from build123d import *

# Parameters (mm, degrees)
SKETCH1_R           = 2.1
SKETCH1_W           = 56
SKETCH1_H           = 115.35
SKETCH1_R_2         = 1.55
BOSS_EXTRUDE1_DEPTH = 3.175
FILLET1_R           = 4
SKETCH10_R          = 2.25
BOSS_EXTRUDE2_DEPTH = 3.175
CIRPATTERN4_COUNT   = 4


with BuildPart() as part:
    # Sketch1 → Boss-Extrude1 (new body)
    with BuildSketch(Plane.XY):
        Polygon((0, 163), (0, 0), (-163, 0), (-163, -17), (-180, -17), (-180, -123), (-163, -123), (-163, -140), (0, -140), (0, -303), (17, -303), (17, -320), (123, -320), (123, -303), (140, -303), (140, -140), (303, -140), (303, -123), (320, -123), (320, -17), (303, -17), (303, 0), (140, 0), (140, 163), (123, 163), (123, 180), (17, 180), (17, 163), align=None)
        with Locations((7.5, -277.5)):
            Circle(SKETCH1_R, mode=Mode.SUBTRACT)
        with Locations((30, -312.5)):
            Circle(SKETCH1_R, mode=Mode.SUBTRACT)
        with Locations((70, -312.5)):
            Circle(SKETCH1_R, mode=Mode.SUBTRACT)
        with Locations((22.5, -265)):
            Circle(SKETCH1_R, mode=Mode.SUBTRACT)
        with BuildLine():
            Line((51.95, -271), (51.95, -265))
            ThreePointArc((51.95, -265), (54, -262.95), (56.05, -265))
            Line((56.05, -265), (56.05, -271))
            ThreePointArc((56.05, -271), (54, -273.05), (51.95, -271))
        make_face(mode=Mode.SUBTRACT)
        with Locations((7.5, -242.5)):
            Circle(SKETCH1_R, mode=Mode.SUBTRACT)
        with Locations((7.5, -207.5)):
            Circle(SKETCH1_R, mode=Mode.SUBTRACT)
        with Locations((22.5, -240)):
            Circle(SKETCH1_R, mode=Mode.SUBTRACT)
        with Locations((70, -202.325)):
            Rectangle(SKETCH1_W, SKETCH1_H, mode=Mode.SUBTRACT)
        with Locations((-172.5, -110)):
            Circle(SKETCH1_R, mode=Mode.SUBTRACT)
        with Locations((-137.5, -132.5)):
            Circle(SKETCH1_R, mode=Mode.SUBTRACT)
        with Locations((-125, -117.5)):
            Circle(SKETCH1_R, mode=Mode.SUBTRACT)
        with Locations((-102.5, -132.5)):
            Circle(SKETCH1_R, mode=Mode.SUBTRACT)
        with Locations((-100, -117.5)):
            Circle(SKETCH1_R, mode=Mode.SUBTRACT)
        with Locations((-67.5, -132.5)):
            Circle(SKETCH1_R, mode=Mode.SUBTRACT)
        with BuildLine():
            ThreePointArc((56.05, -139.65), (54, -141.7), (51.95, -139.65))
            Line((51.95, -139.65), (51.95, -133.65))
            ThreePointArc((51.95, -133.65), (54, -131.6), (56.05, -133.65))
            Line((56.05, -133.65), (56.05, -139.65))
        make_face(mode=Mode.SUBTRACT)
        with Locations((8.5, -86)):
            Circle(SKETCH1_R_2, mode=Mode.SUBTRACT)
        with Locations((110, -312.5)):
            Circle(SKETCH1_R, mode=Mode.SUBTRACT)
        with BuildLine():
            ThreePointArc((83.95, -265), (86, -262.95), (88.05, -265))
            Line((88.05, -265), (88.05, -271))
            ThreePointArc((88.05, -271), (86, -273.05), (83.95, -271))
            Line((83.95, -271), (83.95, -265))
        make_face(mode=Mode.SUBTRACT)
        with Locations((132.5, -277.5)):
            Circle(SKETCH1_R, mode=Mode.SUBTRACT)
        with Locations((117.5, -265)):
            Circle(SKETCH1_R, mode=Mode.SUBTRACT)
        with Locations((132.5, -242.5)):
            Circle(SKETCH1_R, mode=Mode.SUBTRACT)
        with Locations((117.5, -240)):
            Circle(SKETCH1_R, mode=Mode.SUBTRACT)
        with Locations((132.5, -207.5)):
            Circle(SKETCH1_R, mode=Mode.SUBTRACT)
        with BuildLine():
            Line((88.05, -133.65), (88.05, -139.65))
            ThreePointArc((88.05, -139.65), (86, -141.7), (83.95, -139.65))
            Line((83.95, -139.65), (83.95, -133.65))
            ThreePointArc((83.95, -133.65), (86, -131.6), (88.05, -133.65))
        make_face(mode=Mode.SUBTRACT)
        with Locations((131.5, -86)):
            Circle(SKETCH1_R_2, mode=Mode.SUBTRACT)
        with Locations((207.5, -132.5)):
            Circle(SKETCH1_R, mode=Mode.SUBTRACT)
        with Locations((242.5, -132.5)):
            Circle(SKETCH1_R, mode=Mode.SUBTRACT)
        with Locations((277.5, -132.5)):
            Circle(SKETCH1_R, mode=Mode.SUBTRACT)
        with Locations((240, -117.5)):
            Circle(SKETCH1_R, mode=Mode.SUBTRACT)
        with Locations((265, -117.5)):
            Circle(SKETCH1_R, mode=Mode.SUBTRACT)
        with Locations((312.5, -110)):
            Circle(SKETCH1_R, mode=Mode.SUBTRACT)
        with Locations((312.5, -70)):
            Circle(SKETCH1_R, mode=Mode.SUBTRACT)
        with Locations((-172.5, -70)):
            Circle(SKETCH1_R, mode=Mode.SUBTRACT)
        with Locations((-172.5, -30)):
            Circle(SKETCH1_R, mode=Mode.SUBTRACT)
        with Locations((-125, -22.5)):
            Circle(SKETCH1_R, mode=Mode.SUBTRACT)
        with Locations((-100, -22.5)):
            Circle(SKETCH1_R, mode=Mode.SUBTRACT)
        with Locations((-137.5, -7.5)):
            Circle(SKETCH1_R, mode=Mode.SUBTRACT)
        with Locations((-102.5, -7.5)):
            Circle(SKETCH1_R, mode=Mode.SUBTRACT)
        with Locations((-67.5, -7.5)):
            Circle(SKETCH1_R, mode=Mode.SUBTRACT)
        with Locations((8.5, -54)):
            Circle(SKETCH1_R_2, mode=Mode.SUBTRACT)
        with Locations((7.5, 67.5)):
            Circle(SKETCH1_R, mode=Mode.SUBTRACT)
        with Locations((7.5, 102.5)):
            Circle(SKETCH1_R, mode=Mode.SUBTRACT)
        with Locations((22.5, 100)):
            Circle(SKETCH1_R, mode=Mode.SUBTRACT)
        with Locations((7.5, 137.5)):
            Circle(SKETCH1_R, mode=Mode.SUBTRACT)
        with Locations((22.5, 125)):
            Circle(SKETCH1_R, mode=Mode.SUBTRACT)
        with Locations((30, 172.5)):
            Circle(SKETCH1_R, mode=Mode.SUBTRACT)
        with Locations((70, 172.5)):
            Circle(SKETCH1_R, mode=Mode.SUBTRACT)
        with Locations((131.5, -54)):
            Circle(SKETCH1_R_2, mode=Mode.SUBTRACT)
        with Locations((207.5, -7.5)):
            Circle(SKETCH1_R, mode=Mode.SUBTRACT)
        with Locations((240, -22.5)):
            Circle(SKETCH1_R, mode=Mode.SUBTRACT)
        with Locations((242.5, -7.5)):
            Circle(SKETCH1_R, mode=Mode.SUBTRACT)
        with Locations((265, -22.5)):
            Circle(SKETCH1_R, mode=Mode.SUBTRACT)
        with Locations((277.5, -7.5)):
            Circle(SKETCH1_R, mode=Mode.SUBTRACT)
        with Locations((312.5, -30)):
            Circle(SKETCH1_R, mode=Mode.SUBTRACT)
        with Locations((132.5, 67.5)):
            Circle(SKETCH1_R, mode=Mode.SUBTRACT)
        with Locations((117.5, 100)):
            Circle(SKETCH1_R, mode=Mode.SUBTRACT)
        with Locations((132.5, 102.5)):
            Circle(SKETCH1_R, mode=Mode.SUBTRACT)
        with Locations((117.5, 125)):
            Circle(SKETCH1_R, mode=Mode.SUBTRACT)
        with Locations((132.5, 137.5)):
            Circle(SKETCH1_R, mode=Mode.SUBTRACT)
        with Locations((110, 172.5)):
            Circle(SKETCH1_R, mode=Mode.SUBTRACT)
    extrude(amount=BOSS_EXTRUDE1_DEPTH)

    # Fillet1
    fillet1_edges = [part.edges().sort_by_distance(p)[0] for p in [
        (17, -303, 1.5875),
        (0, -140, 1.5875),
        (-163, -123, 1.5875),
        (-163, -17, 1.5875),
        (0, 0, 1.5875),
        (17, 163, 1.5875),
        (123, 163, 1.5875),
        (140, 0, 1.5875),
        (303, -17, 1.5875),
        (303, -123, 1.5875),
        (140, -140, 1.5875),
        (123, -303, 1.5875),
    ]]
    fillet(fillet1_edges, radius=FILLET1_R)

    # Sketch10 → Boss-Extrude2 (add)
    with BuildSketch(Plane.XY):
        Polygon((-127.279220614, -140), (0, -267.279220614), (0, -140), align=None)
        with Locations((-70.710678119, -182.426406871)):
            Circle(SKETCH10_R, mode=Mode.SUBTRACT)
        with Locations((-42.426406871, -210.710678119)):
            Circle(SKETCH10_R, mode=Mode.SUBTRACT)
        with Locations((-63.639610307, -175.355339059)):
            Circle(SKETCH10_R, mode=Mode.SUBTRACT)
        with Locations((-35.355339059, -203.639610307)):
            Circle(SKETCH10_R, mode=Mode.SUBTRACT)
    boss_extrude2 = extrude(amount=BOSS_EXTRUDE2_DEPTH)

    # CirPattern4: Boss-Extrude2 ×4 about axis
    cirpattern4_axis = Axis((70, -70, 0), (0, 0, 1))
    for i in range(1, CIRPATTERN4_COUNT):
        add(boss_extrude2.rotate(cirpattern4_axis, i * 360 / CIRPATTERN4_COUNT))


solid = part.part
Could you check a few things on this model? Use its own coordinates, in mm. Give positions to 0.01 mm unless a question says otherwise; leave off trailing zeros. Order: outer loops, then holes, each group sorted by start corner. A loop starts at its lowest first (then second) coordinate and runs counter-clockwise, first axis right, second up.
1. Suppose I cut it at D-D (x = -19). Write out the boundary of the cut face in (y, z) (3 decimals), plus the area to 3 significant figures.
Answers below:
outline: (-248.279, 0) - (108.279, 0) - (108.279, 3.175) - (-248.279, 3.175) - close
area: 1,130 mm2
2. Suppose I cut it at B-B (z = 1.7). State how many separate pieces and enclosed holes the cut face has, plus the area to 3 significant figures.
Answers below:
separate pieces: 1
enclosed holes: 77
area: 143,000 mm2
3. Suppose I cut it at C-C (x = 147). Write out the boundary of the cut face in (y, z) (3 decimals), plus the area to 3 significant figures.
Answers below:
outline: (-260.279, 0) - (120.279, 0) - (120.279, 3.175) - (-260.279, 3.175) - close
area: 1,210 mm2
4. I need wall thicknesses on L1, parallel to X at y = -86, z = 2.4; L2, parallel to Y at x = 110, z = 2.2; L3, parallel to X at y = 172.5, z = 1.8. Which ranges of each line are inside material? Lowest first, please.
Answers below:
L1: x = -180 to 6.95, 10.05 to 129.95, 133.05 to 320
L2: y = -320 to -314.6, -310.4 to 170.4, 174.6 to 180
L3: x = 17 to 27.9, 32.1 to 67.9, 72.1 to 107.9, 112.1 to 123
5. For pin 1 (1.5 mm diameter, centred on y = 89.5, z = 2.5, fed in from +X); pin 2 (6 mm diameter, centred on x = -90.5, y = 20, fed in from -Z); pin 3 (2.5 mm diameter, centred on x = -125, y = -117.5, fed in from +Z); pin 4 (1.6 mm diameter, centred on x = 316.5, z = 1, fed in from -Y), each with a flat end and sliding along its axis, tell me the tip position at first contact or that it passes through.
Answers below:
pin 1: stops at x = 178.53
pin 2: stops at z = 0
pin 3: passes through
pin 4: stops at y = -123
6. Suppose I cut it at A-A (y = -229.5). Write out the boundary of the cut face in (x, z) (3 decimals).
Answers below:
outline: (-37.779, 0) - (42, 0) - (42, 3.175) - (-37.779, 3.175) - close; (98, 0) - (177.779, 0) - (177.779, 3.175) - (98, 3.175) - close
